Job drawing, mm, ordinate dimensions from the low corner. One solid piece. Give positions to 0.01 mm unless a question says otherwise; leave off trailing zeros. Loops run counter-clockwise (first coordinate to the right, second up) from the corner with the lowest first, then second, coordinate; pieces in that order, holes last. Notation, with made-up numbers: (66, -29) - (115, -29) arc R21 ccw to (115, -11) - close; hole circle Ø11 at (56.5, 29.5). An arc over 180 degrees is marked (long way). Answer as CSV lines item,"result". Start each with the question number.
Item 1: Pin check, flat tips, straight feed: pin 1 (1.6 mm diameter, centred on x = 105, z = 55, fed in from -Y); pin 2 (3 mm diameter, centred on x = 92, y = 4, fed in from +Z); pin 3 (3 mm diameter, centred on x = 55, z = 105, fed in from +Y); pin 4 (1.5 mm diameter, centred on y = 1, z = 27, fed in from -X). Stop position of each tip, or through.
Item 2: Saw through at A-A on x = 67.5. Give the cut face in (y, z), plus the area to 3 significant figures.
Item 3: Saw through at C-C on y = 1.85. Give the cut face in (x, z), plus the area to 3 significant figures.
Item 4: Saw through at B-B on z = 48. Give the cut face in (x, y).
Item 5: Drill centre lines: L1, parallel to Z at x = 55, y = 1.6; L2, parallel to Y at x = 37.5, z = 11.5; L3, parallel to X at y = 1.85, z = 105. Where is each one in solid material? Low to high. Write a range as from..to.
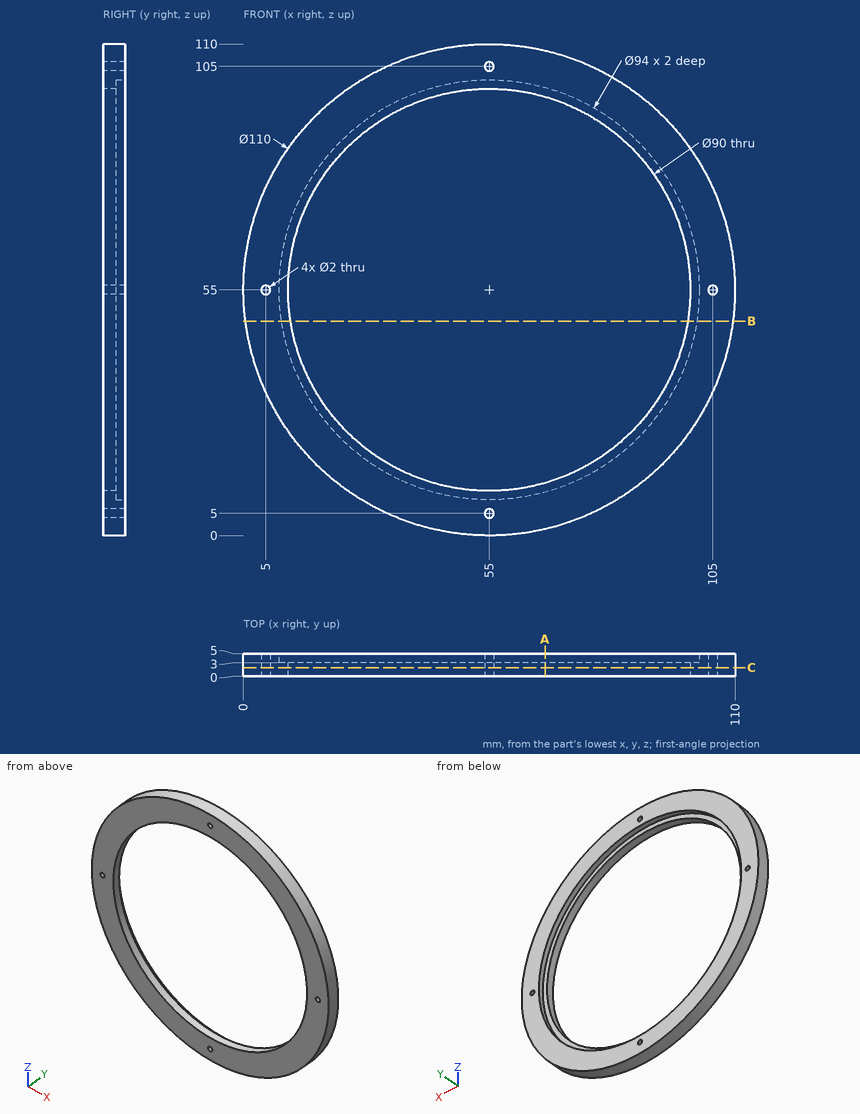
Responses:
1,pin 1,"through"
1,pin 2,"z = 97.01"
1,pin 3,"y = 5"
1,pin 4,"x = 7.23"
2,outline,"(0, 1.44) - (5, 1.44) - (5, 9.69) - (3, 9.69) - (3, 11.77) - (0, 11.77) - close; (0, 98.23) - (3, 98.23) - (3, 100.31) - (5, 100.31) - (5, 108.56) - (0, 108.56) - close"
2,area,"95.0 mm2"
3,outline,"circle Ø110 at (55, 55); hole circle Ø2 at (5, 55); hole circle Ø90 at (55, 55); hole circle Ø2 at (55, 5); hole circle Ø2 at (55, 105); hole circle Ø2 at (105, 55)"
3,area,"3,130 mm2"
4,outline,"(0.45, 0) - (10.55, 0) - (10.55, 3) - (8.52, 3) - (8.52, 5) - (0.45, 5) - close; (99.45, 0) - (109.55, 0) - (109.55, 5) - (101.48, 5) - (101.48, 3) - (99.45, 3) - close"
5,L1,"0..4, 6..10, 100..104, 106..110"
5,L2,"0..3"
5,L3,"32.09..54, 56..77.91"
